The listing builds one solid part. Answer for the finished solid, in the listing's coordinates (mm). Face numbers are marked on the shaded views. Give positions to 0.01 mm unless a question says otherwise; leave off trailing zeros. Order: outer loops, then holes, each group sorted by start corner. A loop starts at its lowest first (then second) coordinate and runs counter-clockwise, first axis right, second up.
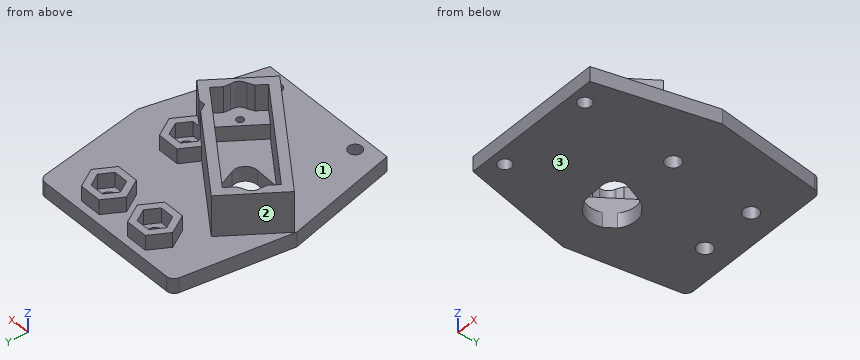
Autodesk Inventor part; units mm, degrees
ref_plane "Work Plane1" through (0, 176.5909, 4) normal (1, 0, 0) x (0, 0, -1)
ref_plane "YZ Plane" through (0, 0, 0) normal (1, 0, 0) x (0, 1, 0)
ref_plane "XZ Plane" through (0, 0, 0) normal (0, 1, 0) x (-1, 0, 0)
sketch "Sketch1" plane through (0, 0, 0) normal (0, 0, 1) x (1, 0, 0)
  circle A0 centre (-7.5, 23) radius 2
  circle A1 centre (-9.9, 0) radius 2
  line L0 (0, 30) -> (-21.5, 30)
  line L1 (-21.5, 30) -> (-25.9, 0)
  line L2 (-25.9, 0) -> (-19, -30)
  line L3 (-19, -30) -> (0, -30)
  line L4 (0, -30) -> (0, 30) construction
  line L5 (-9.9, 0) -> (0, 0)
  line L6 (0, 30) -> (21.5, 30)
  line L7 (21.5, 30) -> (25.9, 0)
  line L8 (25.9, 0) -> (19, -30)
  line L9 (19, -30) -> (0, -30)
  circle A2 centre (7.5, 23) radius 2
  circle A3 centre (9.9, 0) radius 2
  dimension "d0" = 4
  dimension "d1" = 4
  dimension "d3" = 14
  dimension "d6" = 16
  dimension "d7" = 7
  dimension "d8" = 19
  dimension "d9" = 30
  dimension "d10" = 30
  dimension "d11" = 19
  dimension "d12" = 21.5
  dimension "d13" = 4
  dimension "d14" = 7
  dimension "d15" = 7.5
  dimension "d16" = 30
  dimension "d17" = 30
  dimension "d18" = 4
  dimension "d20" = 16
  dimension "d47" = 9.9
  dimension "d79" = 9.9
  dimension "d98" = 7.5
extrude "Extrusion1" add sketch "Sketch1" along normal blind 4
fillet "Fillet1" radius 2 2 edges at (-21.5, 30, 2) (21.5, 30, 2)
ref_plane "Work Plane1" through (0, 176.5909, 4) normal (1, 0, 0) x (0, 0, -1)
sketch "Sketch2" plane through (0, 0, 4) normal (0, 0, 1) x (1, 0, 0)
  circle A0 centre (-9.9, 0) radius 2
  line L0 (-15.7104, 14.6282) -> (15.1061, -6.9498)
  line L1 (15.1061, -6.9498) -> (5.1832, -21.1211)
  line L2 (5.1832, -21.1211) -> (-25.6333, 0.4569)
  line L3 (-25.6333, 0.4569) -> (-15.7104, 14.6282)
  line L4 (-20.6718, 7.5425) -> (10.1447, -14.0354) construction
  line L5 (-15.0965, 11.1464) -> (11.6243, -7.5637)
  line L6 (11.6243, -7.5637) -> (4.5693, -17.6393)
  line L7 (4.5693, -17.6393) -> (-22.1515, 1.0708)
  line L8 (-22.1515, 1.0708) -> (-15.0965, 11.1464)
  line L9 (-15.0965, 11.1464) -> (-11.3693, 8.5366)
  line L10 (-11.3693, 8.5366) -> (-18.4243, -1.539)
  line L11 (-18.4243, -1.539) -> (-22.1515, 1.0708)
  line L12 (-22.1515, 1.0708) -> (-15.0965, 11.1464)
  line L13 (4.5693, -17.6393) -> (0.8421, -15.0295)
  line L14 (7.8971, -4.9539) -> (11.6243, -7.5637)
  line L15 (11.6243, -7.5637) -> (4.5693, -17.6393)
  line L16 (0, 42) -> (0, -42)
  line L17 (0.8421, -15.0295) -> (7.8971, -4.9539)
  dimension "d34" = 37.62
  dimension "d35" = 17.3
  dimension "d36" = 2.5
  dimension "d37" = 2.5
  dimension "d38" = 2.5
  dimension "d40" = 2.5
  dimension "d42" = 4.55
  dimension "d44" = 55
  dimension "d45" = 6.15
  dimension "d46" = 4.55
  dimension "d78" = 6.1
extrude "Extrusion2" add sketch "Sketch2" along normal blind 4 contours L10 L7 L8 L5 | L5 L6 L7 L17
extrude "Extrusion3" add sketch "Sketch2" along normal blind 11 contours L0 L16 L5 L8 L7 L2 L3 | L0 L1 L2 L16 L7 L6 L5
sketch "Sketch3" plane through (0, 0, 15) normal (0, 0, 1) x (1, 0, 0)
  line L0 (-15.7104, 14.6282) -> (-25.6333, 0.4569)
  line L1 (-25.6333, 0.4569) -> (5.1832, -21.1211)
  line L2 (5.1832, -21.1211) -> (15.1061, -6.9498)
  line L3 (15.1061, -6.9498) -> (-15.7104, 14.6282)
  line L4 (-15.0965, 11.1464) -> (11.6243, -7.5637)
  line L5 (11.6243, -7.5637) -> (4.5693, -17.6393)
  line L6 (4.5693, -17.6393) -> (-22.1515, 1.0708)
  line L7 (-22.1515, 1.0708) -> (-15.0965, 11.1464)
  line L8 (-18.624, 6.1086) -> (8.0968, -12.6015) construction
  circle A0 centre (-16.5269, 4.6402) radius 0.95
  circle A1 centre (5.9997, -11.1331) radius 0.95
  line L9 (-18.4243, -1.539) -> (-11.3693, 8.5366)
  line L10 (7.8971, -4.9539) -> (0.8421, -15.0295)
  arc A2 (-15.8617, 3.9621) -> (-17.3097, 7.9855) centre (-17.8048, 5.535) ccw construction
  arc A3 (6.7825, -14.4784) -> (9.411, -10.7246) centre (7.2776, -12.0279) ccw
  arc A4 (-19.9382, 4.2317) -> (-15.8617, 3.9621) centre (-17.8048, 5.535) ccw construction
  arc A5 (-17.3097, 7.9855) -> (-19.9382, 4.2317) centre (-17.8048, 5.535) ccw
  arc A6 (5.1349, -10.7399) -> (6.7825, -14.4784) centre (7.2776, -12.0279) ccw construction
  arc A7 (9.411, -10.7246) -> (5.1349, -10.7399) centre (7.2776, -12.0279) ccw construction
  point P0 (0, 0)
  dimension "d52" = 1.9
  dimension "d53" = 1.9
  dimension "d54" = 1.99
  dimension "d55" = 1.99
  dimension "d56" = 5
  dimension "d57" = 3.5
  dimension "d58" = 5
  dimension "d59" = 3.5
extrude "Extrusion4" cut sketch "Sketch3" against normal up to surface (7 mm away) contours L7 A5 | A3 L5
chamfer "Chamfer1" distance 1 angle 45 4 edges at (-17.3097, 7.9855, 11.5) (-19.9382, 4.2317, 11.5) (6.7825, -14.4784, 11.5) (9.411, -10.7246, 11.5)
extrude "Extrusion5" cut sketch "Sketch3" against normal blind 14 contours A0 | A1
sketch "Sketch4" plane through (0, 0, 4) normal (0, 0, 1) x (1, 0, 0)
  circle A0 centre (-9.9, 0) radius 2
  line L0 (-18.4243, -1.539) -> (-11.3693, 8.5366)
  line L1 (-18.4243, -1.539) -> (0.8421, -15.0295)
  line L2 (0.8421, -15.0295) -> (7.8971, -4.9539)
  line L3 (7.8971, -4.9539) -> (-11.3693, 8.5366)
  line L4 (-11.3693, 8.5366) -> (-18.4243, -1.539)
  circle A1 centre (-9.9, 0) radius 2
  arc A2 (-7.2134, -5.6984) -> (-4.0762, 2.4029) centre (-9.9, 0) ccw construction
  arc A3 (-5.241, -6.5026) -> (-2.1961, -2.154) centre (-5.108, -3.3554) ccw
  line L5 (-4.0762, 2.4029) -> (-2.1961, -2.154)
  line L6 (-10.1661, -6.2944) -> (-5.241, -6.5026)
  line L7 (-14.8968, 3.4988) -> (4.3696, -9.9917) construction
  arc A4 (-10.1661, -6.2944) -> (-7.2134, -5.6984) centre (-9.9, 0) ccw construction
  arc A5 (-7.2134, -5.6984) -> (-5.241, -6.5026) centre (-5.108, -3.3554) ccw construction
  arc A6 (-4.0762, 2.4029) -> (-10.1661, -6.2944) centre (-9.9, 0) ccw
  arc A7 (-2.1961, -2.154) -> (-7.2134, -5.6984) centre (-5.108, -3.3554) ccw construction
  point P0 (0, 0)
  point P1 (-5.2531, 4.254)
  point P2 (-7.4919, 5.8216)
  point P3 (-13.9936, 4.7888)
  point P4 (-15.8001, 2.2088)
  point P5 (-14.5469, -4.254)
  point P6 (-12.3081, -5.8216)
  dimension "d73" = 12.6
  dimension "d74" = 6.3
  dimension "d75" = 5.85
extrude "Extrusion6" cut sketch "Sketch4" against normal through all contours L0 A6 L3 L5 A3 L6 L1
sketch "Sketch5" plane through (0, 0, 4) normal (0, 0, 1) x (1, 0, 0)
  circle A0 centre (-7.5, 23) radius 2
  circle A1 centre (7.5, 23) radius 2
  circle A2 centre (9.9, 0) radius 2
  line L0 (-5.6236, 26.25) -> (-3.7472, 23)
  line L1 (-3.7472, 23) -> (-5.6236, 19.75)
  line L2 (-5.6236, 19.75) -> (-9.3764, 19.75)
  line L3 (-9.3764, 19.75) -> (-11.2528, 23)
  line L4 (-11.2528, 23) -> (-9.3764, 26.25)
  line L5 (-9.3764, 26.25) -> (-5.6236, 26.25)
  line L6 (9.3764, 26.25) -> (11.2528, 23)
  line L7 (11.2528, 23) -> (9.3764, 19.75)
  line L8 (9.3764, 19.75) -> (5.6236, 19.75)
  line L9 (5.6236, 19.75) -> (3.7472, 23)
  line L10 (3.7472, 23) -> (5.6236, 26.25)
  line L11 (5.6236, 26.25) -> (9.3764, 26.25)
  line L12 (11.7764, 3.25) -> (13.6528, 0)
  line L13 (13.6528, 0) -> (11.7764, -3.25)
  line L14 (11.7764, -3.25) -> (8.0236, -3.25)
  line L15 (8.0236, -3.25) -> (6.1472, 0)
  line L16 (6.1472, 0) -> (8.0236, 3.25)
  line L17 (8.0236, 3.25) -> (11.7764, 3.25)
  line L18 (-4.6132, 28) -> (-1.7265, 23)
  line L19 (-1.7265, 23) -> (-4.6132, 18)
  line L20 (-4.6132, 18) -> (-10.3868, 18)
  line L21 (-10.3868, 18) -> (-13.2735, 23)
  line L22 (-13.2735, 23) -> (-10.3868, 28)
  line L23 (-10.3868, 28) -> (-4.6132, 28)
  line L24 (4.6132, 18) -> (10.3868, 18)
  line L25 (10.3868, 18) -> (13.2735, 23)
  line L26 (13.2735, 23) -> (10.3868, 28)
  line L27 (10.3868, 28) -> (4.6132, 28)
  line L28 (4.6132, 28) -> (1.7265, 23)
  line L29 (1.7265, 23) -> (4.6132, 18)
  line L30 (12.7868, 5) -> (15.6735, 0)
  line L31 (15.6735, 0) -> (12.7868, -5)
  line L32 (12.7868, -5) -> (7.9629, -5)
  line L33 (7.0132, -5) -> (6.3688, -3.8838) construction
  line L34 (4.1265, 0) -> (7.0132, 5)
  line L35 (7.0132, 5) -> (12.7868, 5)
  line L36 (-15.0965, 11.1464) -> (11.6243, -7.5637)
  line L37 (6.3688, -3.8838) -> (4.1265, 0)
  line L38 (7.9629, -5) -> (7.0132, -5) construction
  point P0 (0, 0)
  point P1 (9.9, 3.25)
  dimension "d80" = 6.5
  dimension "d81" = 6.5
  dimension "d82" = 6.5
  dimension "d85" = 10
  dimension "d86" = 10
  dimension "d87" = 10
extrude "Extrusion7" cut sketch "Sketch5" along normal through all contours A2 | L12 L13 L14 L15 L16 L17
extrude "Extrusion8" add sketch "Sketch5" along normal blind 4 contours L18 L19 L20 L21 L22 L23 | L29 L28 L27 L26 L25 L24 | L30 L31 L32 L36 L37 L34 L35
sketch "Sketch6" plane through (0, 0, 0) normal (0, 0, -1) x (-1, 0, 0)
  circle A0 centre (-13, -26.4) radius 1.75
  circle A1 centre (13, -26.4) radius 1.75
  line L0 (19, -30) -> (-19, -30)
  point P0 (0, 0)
  dimension "d90" = 3.5
  dimension "d91" = 3.5
  dimension "d92" = 26
  dimension "d93" = 13
  dimension "d94" = 3.6
  dimension "d95" = 3.6
extrude "Extrusion9" cut sketch "Sketch6" against normal through all
equation "\"d1\" = d0"
equation "\"d11\" = d8"
equation "\"d13\" = d0"
equation "\"d14\" = d7"
equation "\"d18\" = d0"
equation "\"d47\" = d79"
equation "\"d81\" = d80"
equation "\"d86\" = d85"
equation "\"d87\" = d86"
equation "\"d95\" = d94"
properties part number "head"
1) Find section D-D (z = 2.25). Count the separate pieces of the cut face and the enclosed holes in it, then the cut area to 3 significant figures.
Geometry says:
separate pieces: 1
enclosed holes: 8
area: 2,560 mm2
2) Find section A-A (z = 10). Write down the section's boundary in (x, y).
Geometry says:
outline: (-25.63, 0.46) - (5.18, -21.12) - (15.11, -6.95) - (9.82, -3.25) - (8.02, -3.25) - (6.8, -1.14) - (-15.71, 14.63) - close; hole (-22.15, 1.07) - (4.57, -17.64) - (6.21, -15.3) - (7.78, -14.48) arc R2.5 ccw to (9.75, -11.66) - (9.98, -9.91) - (11.62, -7.56) - (-15.1, 11.15) - (-16.74, 8.8) - (-18.31, 7.98) arc R2.5 ccw to (-20.28, 5.17) - (-20.51, 3.41) - close
3) For a pull along Y with two mould halves and no side action, classify the marked faces 1, 2 and 3 as +Y half, -Y half, draft (parallel to the pull), parting line (faces both ways), or undercut.
Geometry says:
face 1: undercut
face 2: +Y half
face 3: draft
4) Straight lines are drawn through the part: probe 1 along Y at (x, z) = (13, 2.3); probe 2 along Y at (x, z) = (-13, 1.75); probe 3 along Y at (x, z) = (7.5, 1.2). For each, find the intervals that lie inside material, in ascending order.
Geometry says:
probe 1: y = -30 to -28.15, -24.65 to 30
probe 2: y = -30 to -28.15, -24.65 to -5.34, 5.48 to 30
probe 3: y = -30 to 21, 25 to 30
5) Find section C-C (y = -9). Write down the section's boundary in (x, z).
Geometry says:
outline: (-23.83, 0) - (23.83, 0) - (23.83, 4) - (13.67, 4) - (13.67, 15) - (10.62, 15) - (10.62, 8) - (5.06, 8) - (5.06, 4) - (-7.77, 4) - (-7.77, 15) - (-12.13, 15) - (-12.13, 4) - (-23.83, 4) - close
6) Given P1, Ø4, axis at y = -5, z = 5, coming from the -X side; P2, Ø3.5, axis at x = 8, y = 0.5, coming from the +Z side; P3, Ø2, axis at x = -9, z = 8, coming from the -Y side, each flat-ended and moving along its own axis, determine where each tip first touches the part or whether it passes through.
Geometry says:
P1: stops at x = -25.15
P2: stops at z = 8
P3: stops at y = -11.89
7) Find section B-B (x = -8.5). Write down the section's boundary in (y, z), then the cut area to 3 significant figures.
Geometry says:
outline: (-30, 0) - (-6.36, 0) - (-6.36, 4) - (-8.49, 4) - (-8.49, 15) - (-11.54, 15) - (-11.54, 4) - (-30, 4) - close; (6.14, 0) - (21.27, 0) - (21.27, 4) - (19.75, 4) - (19.75, 8) - (18, 8) - (18, 4) - (9.58, 4) - (9.58, 15) - (6.53, 15) - (6.53, 4) - (6.14, 4) - close; (24.73, 0) - (30, 0) - (30, 4) - (28, 4) - (28, 8) - (26.25, 8) - (26.25, 4) - (24.73, 4) - close
area: 257 mm2
